from build123d import *

# Parameters (mm, degrees)
ESQUISSE1_R        = 26
ESQUISSE1_R_2      = 2
ESQUISSE1_R_3      = 11
BOSS_EXTRU_1_DEPTH = 0.8
ESQUISSE2_R        = 13
ESQUISSE2_R_2      = 11
BOSS_EXTRU_2_DEPTH = 1.4


with BuildPart() as part:
    # Esquisse1 → Boss.-Extru.1 (new body)
    with BuildSketch(Plane.XY):
        Circle(ESQUISSE1_R)
        with Locations((0, 22)):
            Circle(ESQUISSE1_R_2, mode=Mode.SUBTRACT)
        with Locations((19.053058883, 11.000866025)):
            Circle(ESQUISSE1_R_2, mode=Mode.SUBTRACT)
        with Locations((19.054058883, -10.999133975)):
            Circle(ESQUISSE1_R_2, mode=Mode.SUBTRACT)
        with Locations((0.002, -22)):
            Circle(ESQUISSE1_R_2, mode=Mode.SUBTRACT)
        with Locations((-19.051058883, -11.000866025)):
            Circle(ESQUISSE1_R_2, mode=Mode.SUBTRACT)
        with Locations((-19.052058883, 10.999133975)):
            Circle(ESQUISSE1_R_2, mode=Mode.SUBTRACT)
        Circle(ESQUISSE1_R_3, mode=Mode.SUBTRACT)
    extrude(amount=BOSS_EXTRU_1_DEPTH)

    # Esquisse2 → Boss.-Extru.2 (add)
    with BuildSketch(Plane.XY.offset(0.8)):
        Circle(ESQUISSE2_R)
        Circle(ESQUISSE2_R_2, mode=Mode.SUBTRACT)
    extrude(amount=BOSS_EXTRU_2_DEPTH)


solid = part.part
Could you check a few things on this model? Use its own coordinates, in mm. A direction names the side the tool comes from. Round coordinates to 2 decimals unless told otherwise and drop trailing zeros. Loops run counter-clockwise (first coordinate to the right, second up) from the corner with the lowest first, then second, coordinate; pieces in that order, holes last. Notation, with made-up numbers: (-32, 2.5) -> (14, 2.5) arc R21 cw to (14, 36.5) -> close; hole circle Ø9 at (78.5, 41). An arc over 180 degrees is marked (long way). Use CSV: the item, a comma, the result in double quotes.
(1) If I drill on probe 1 along Y at (x, z) = (0, 0.1); probe 2 along Y at (x, z) = (0.5, 1.05); probe 3 along Y at (x, z) = (-19.5, 0.25), over which ranges is the centre line in solid material (lowest first)? Write a range as [from, to].
Return value:
probe 1,"y = [-26, -24], [-20, -11], [11, 20], [24, 26]"
probe 2,"y = [-12.99, -10.99], [10.99, 12.99]"
probe 3,"y = [-17.2, -12.95], [-9.05, 9.05], [12.95, 17.2]"
(2) Suppose I cut it at A-A on x = 0. Write out the boundary of the cut face in (y, z), plus the area to 3 significant figures.
Return value:
outline,"(-26, 0) -> (-24, 0) -> (-24, 0.8) -> (-26, 0.8) -> close; (-20, 0) -> (-11, 0) -> (-11, 2.2) -> (-13, 2.2) -> (-13, 0.8) -> (-20, 0.8) -> close; (11, 0) -> (20, 0) -> (20, 0.8) -> (13, 0.8) -> (13, 2.2) -> (11, 2.2) -> close; (24, 0) -> (26, 0) -> (26, 0.8) -> (24, 0.8) -> close"
area,"23.2 mm²"
(3) Suppose I cut it at C-C on x = 19. Write out the boundary of the cut face in (y, z), plus the area to 3 significant figures.
Return value:
outline,"(-17.75, 0) -> (-13, 0) -> (-13, 0.8) -> (-17.75, 0.8) -> close; (-9, 0) -> (9, 0) -> (9, 0.8) -> (-9, 0.8) -> close; (13, 0) -> (17.75, 0) -> (17.75, 0.8) -> (13, 0.8) -> close"
area,"22.0 mm²"
(4) Will these pins go through, and if not, where does the flat tip stop? pin 1 Ø3.5 at (x, y) = (-19.05, 11) entering from -Z; pin 2 Ø5 at (x, y) = (13.5, -15) entering from +Z; pin 3 Ø4 at (x, y) = (0.5, -9.5) entering from -Z.
Return value:
pin 1,"passes through"
pin 2,"stops at z = 0.8"
pin 3,"stops at z = 0"
(5) Suppose I cut it at B-B on y = 0. Write out the boundary of the cut face in (x, z).
Return value:
outline,"(-26, 0) -> (-11, 0) -> (-11, 2.2) -> (-13, 2.2) -> (-13, 0.8) -> (-26, 0.8) -> close; (11, 0) -> (26, 0) -> (26, 0.8) -> (13, 0.8) -> (13, 2.2) -> (11, 2.2) -> close"
(6) For faces 4 (the cylindrical face through (-10.316, -7.91, 1.49)), 5 (the cylindrical face through (-18, -9.3, 0.4)), which set-ups out of +Z, -Z, +X, -X, +Y, -Y let a thin tool reach every point of the face, with its end or its side?
Return value:
face 4,"+Z"
face 5,"+Z, -Z"
(7) If we mould it in two halves opening along X, with no side actions, what happens to faces 1 (the cylindrical face through (-20.633, -15.821, 0.394)), 2 (the cylindrical face through (17.055, 11.089, 0.394)), 3 (the flat face through (-6, 12, 0.8))? For each: +X half, -X half, draft (parallel to the pull), parting line (faces both ways), or undercut.
Return value:
face 1,"parting line"
face 2,"undercut"
face 3,"draft"
(8) Suppose I cut it at D-D on x = 7. Write out the boundary of the cut face in (y, z), plus the area to 3 significant figures.
Return value:
outline,"(-25.04, 0) -> (-8.49, 0) -> (-8.49, 2.2) -> (-10.95, 2.2) -> (-10.95, 0.8) -> (-25.04, 0.8) -> close; (8.49, 0) -> (25.04, 0) -> (25.04, 0.8) -> (10.95, 0.8) -> (10.95, 2.2) -> (8.49, 2.2) -> close"
area,"33.4 mm²"
